Work out the finished part from the listing and answer in its coordinate system (mm). Face numbers are marked on the shaded views. A direction names the side the tool comes from. Round coordinates to 2 decimals unless told otherwise and drop trailing zeros. Order: outer loops, then holes, each group sorted by start corner. A loop starts at its lowest first (then second) coordinate and runs counter-clockwise, first axis right, second up. Notation, with made-up numbers: (64, -23) - (116, -23) arc R21 cw to (116, 13) - close; hole circle Ø10 at (-28.5, -14.75). An arc over 180 degrees is marked (long way). Put each result on its own line as item: value.
```python
from build123d import *
from build123d import SkipClean  # not in build123d's __all__

# Parameters (mm, degrees)
F1_DEPTH = 6.35
F2_W     = 13.3050326258
F2_H     = 13.3050344884
F2_R     = 6.4893385046
F3_DEPTH = 6.35
F4_DEPTH = 25.4
F5_DEPTH = 7.112
F7_DEPTH = 6.35
F8_R     = 3.7056239581
F9_DEPTH = 2.54


# Not quite as in the source:
# - after a boolean that leaves OpenCascade's solid faulty, fix() repairs it


with BuildPart() as f1:
    # F0 (on Front) → F1 (new body)
    with BuildSketch(Plane.XZ):
        with BuildLine():
            ThreePointArc((-31.8034514785, 8.237525334), (-33.7084514785, 11.1474609002), (-31.8034514785, 14.0573964665))
            Line((-31.8034514785, 14.0573964665), (-31.8034514785, 17.5113130534))
            ThreePointArc((-31.8034514785, 17.5113130534), (-37.0227899831, 11.1474609002), (-31.8034514785, 4.7836087471))
            Line((-31.8034514785, 4.7836087471), (-31.8034514785, 8.237525334))
        make_face()
        with BuildLine():
            Line((-31.8034514785, 8.237525334), (-31.8034514785, 14.0573964665))
            ThreePointArc((-31.8034514785, 14.0573964665), (-33.7084514785, 11.1474609002), (-31.8034514785, 8.237525334))
        make_face()
        with BuildLine():
            ThreePointArc((-31.8034514785, 14.0573964665), (-28.7944323584, 13.8038564845), (-27.3584514785, 11.1474609002))
            ThreePointArc((-27.3584514785, 11.1474609002), (-28.7944323584, 8.491065316), (-31.8034514785, 8.237525334))
            Line((-31.8034514785, 8.237525334), (-31.8034514785, 4.7836087471))
            ThreePointArc((-31.8034514785, 4.7836087471), (-26.4182325094, 6.129843232), (-24.0441129739, 11.1474609002))
            ThreePointArc((-24.0441129739, 11.1474609002), (-26.4182325094, 16.1650785684), (-31.8034514785, 17.5113130534))
            Line((-31.8034514785, 17.5113130534), (-31.8034514785, 14.0573964665))
        make_face()
    extrude(amount=F1_DEPTH)

    # F2 (on face) → F3 (join)
    with BuildSketch(Plane.XZ.offset(6.35)):
        with Locations((-30.5656185374, 11.1557710916)):
            Rectangle(F2_W, F2_H)
        with Locations((-30.5334514785, 11.1474609002)):
            Circle(F2_R, mode=Mode.SUBTRACT)
        with Locations((-30.5334514785, 11.1474609002)):
            Circle(F2_R)
        with BuildLine():
            ThreePointArc((-31.8034514785, 14.0573964665), (-27.3584514785, 11.1474609002), (-31.8034514785, 8.237525334))
            Line((-31.8034514785, 8.237525334), (-31.8034514785, 14.0573964665))
        make_face(mode=Mode.SUBTRACT)
    extrude(amount=F3_DEPTH)

    # F0 (on Front) → F4 (cut)
    with BuildSketch(Plane.XZ):
        with BuildLine():
            Line((-31.8034514785, 8.237525334), (-31.8034514785, 14.0573964665))
            ThreePointArc((-31.8034514785, 14.0573964665), (-33.7084514785, 11.1474609002), (-31.8034514785, 8.237525334))
        make_face()
    extrude(amount=F4_DEPTH, mode=Mode.SUBTRACT)

    # F0 (on Front) → F5 (join)
    with BuildSketch(Plane.XZ):
        with BuildLine():
            Line((-31.8034514785, 8.237525334), (-31.8034514785, 14.0573964665))
            ThreePointArc((-31.8034514785, 14.0573964665), (-33.7084514785, 11.1474609002), (-31.8034514785, 8.237525334))
        make_face()
    extrude(amount=F5_DEPTH)

    # F6 (on face) → F7 (join)
    with BuildSketch(Plane(origin=(0, 0, 0), x_dir=(-1, 0, 0), z_dir=(0, 1, 0))):
        with BuildLine():
            ThreePointArc((32.1643167645, 17.4285271033), (27.7190855009, 14.0622502303), (24.1990881726, 9.7377248483))
            ThreePointArc((24.1990881726, 9.7377248483), (29.2426072016, 7.0222894593), (34.9343685496, 6.3784522862))
            ThreePointArc((34.9343685496, 6.3784522862), (34.7517106144, 12.2049013649), (32.1643167645, 17.4285271033))
        make_face()
        with BuildLine():
            Line((31.8034514785, 14.0573964665), (31.8034514785, 8.237525334))
            ThreePointArc((31.8034514785, 8.237525334), (27.3584514785, 11.1474609002), (31.8034514785, 14.0573964665))
        make_face(mode=Mode.SUBTRACT)
    with SkipClean():  # cleaning this boolean's faces spoils the solid; the shape is the same uncleaned
        extrude(amount=F7_DEPTH)

    # F8 (on face) → F9 (join)
    with BuildSketch(Plane(origin=(0, 6.35, 0), x_dir=(-1, 0, 0), z_dir=(0, 1, 0))):
        with Locations((30.5334514785, 11.1474609002)):
            Circle(F8_R)
        with BuildLine():
            ThreePointArc((31.8034514785, 8.237525334), (27.3584514785, 11.1474609002), (31.8034514785, 14.0573964665))
            Line((31.8034514785, 14.0573964665), (31.8034514785, 8.237525334))
        make_face(mode=Mode.SUBTRACT)
        with BuildLine():
            Line((31.8034514785, 8.237525334), (31.8034514785, 14.0573964665))
            ThreePointArc((31.8034514785, 14.0573964665), (27.3584514785, 11.1474609002), (31.8034514785, 8.237525334))
        make_face()
    extrude(amount=F9_DEPTH)

    add(f1.part.fix(), mode=Mode.REPLACE)


solid = f1.part
```
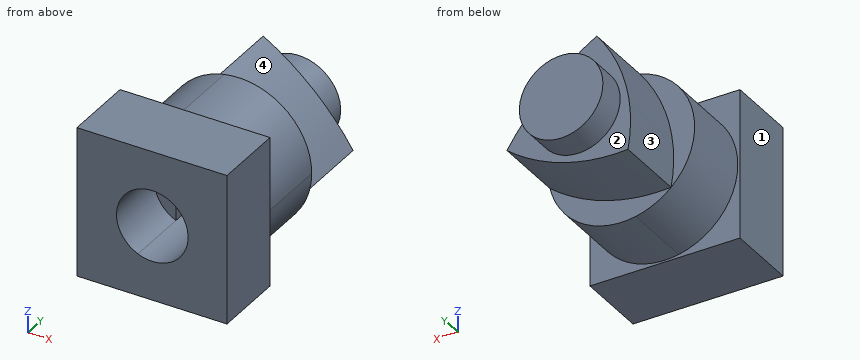
1) A cutting plane is placed at B-B on x = -36. Write down the section's boundary in (y, z).
Findings below:
outline: (-12.7, 4.5) - (-6.35, 4.5) - (-6.35, 7.65) - (0, 7.65) - (0, 14.64) - (-6.35, 14.64) - (-6.35, 17.81) - (-12.7, 17.81) - close
2) Straight lines are drawn through the part: L1, parallel to Y at x = -31.75, z = 11.75; L2, parallel to Y at x = -27.5, z = 8.75; L3, parallel to Z at x = -30, y = -5.5. For each, find the intervals that lie inside material, in ascending order. Write a range as from..to.
Findings below:
L1: y = 6.35..8.89
L2: y = -12.7..6.35
L3: z = 4.68..8.02, 14.28..17.61
3) A cutting plane is placed at A-A on y = 1.5. Write down the section's boundary in (x, z) (3 decimals).
Findings below:
outline: (-34.934, 6.378) arc R15.116 ccw to (-24.199, 9.738) arc R23.342 ccw to (-32.164, 17.429) arc R13.707 ccw to start; hole (-31.803, 8.238) arc R3.175 ccw (long way) to (-31.803, 14.057) - close
4) For the marked faces 1, 2, 3 and 4, determine the directions among +Z, -Z, +X, -X, +Y, -Y from which every point of the face is accessible in a straight line to the end or side of a thin tool.
Findings below:
face 1: +Z, -Z, -X, +Y, -Y
face 2: +Y
face 3: -X, +Y
face 4: +Z, +X, +Y
5) Given pin 1 Ø4 at (x, z) = (-30.5, 12) entering from -Y; pin 2 Ø2 at (y, z) = (5, 15) entering from -X; pin 3 Ø6.5 at (y, z) = (1, 12) entering from +X, each flat-ended and moving along its own axis, determine where each tip first touches the part or whether it passes through.
Findings below:
pin 1: stops at y = -7.11
pin 2: stops at x = -34.17
pin 3: stops at x = -24.04
6) A cutting plane is placed at D-D on y = -5.5. Write down the section's boundary in (x, z) (3 decimals), then the cut area to 3 significant figures.
Findings below:
outline: circle Ø12.979 at (-30.533, 11.147); hole (-31.803, 8.238) arc R3.175 ccw (long way) to (-31.803, 14.057) - close
area: 109 mm2
7) A cutting plane is placed at C-C on z = 8.75. Write down the section's boundary in (x, y) (3 decimals).
Findings below:
outline: (-37.218, -12.7) - (-32.615, -12.7) - (-32.615, -7.112) - (-31.803, -7.112) - (-31.803, 6.35) - (-28.452, 6.35) - (-28.452, -12.7) - (-23.913, -12.7) - (-23.913, -6.35) - (-24.503, -6.35) - (-24.503, 0) - (-25.557, 0) - (-25.557, 6.35) - (-27.708, 6.35) - (-27.708, 8.89) - (-33.359, 8.89) - (-33.359, 6.35) - (-35.163, 6.35) - (-35.163, 0) - (-36.564, 0) - (-36.564, -6.35) - (-37.218, -6.35) - close
